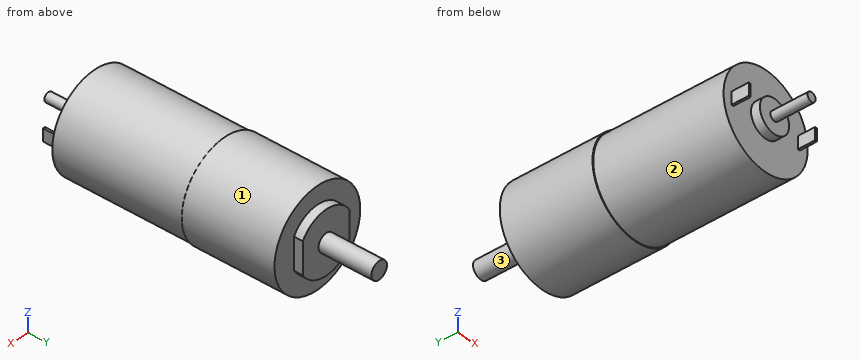
from build123d import *

# Parameters (mm, degrees)
SKETCH2_R           = 10.8
BOSS_EXTRUDE1_DEPTH = 29.5
SKETCH3_R           = 11
BOSS_EXTRUDE2_DEPTH = 21
BOSS_EXTRUDE3_DEPTH = 2
SKETCH5_R           = 2
BOSS_EXTRUDE4_DEPTH = 12
SKETCH6_R           = 3.75
BOSS_EXTRUDE5_DEPTH = 2
SKETCH7_W           = 0.5
SKETCH7_H           = 2.8
BOSS_EXTRUDE6_DEPTH = 3.9
SKETCH8_R           = 1.05
BOSS_EXTRUDE7_DEPTH = 8.4


with BuildPart() as part:
    # Sketch2 → Boss-Extrude1 (new body)
    with BuildSketch(Plane(origin=(0, 0, 0), x_dir=(1, 0, 0), z_dir=(0, 1, 0))):
        with Locations(Location((0, 0, 0), (0, 0, 270))):
            Circle(SKETCH2_R)
    extrude(amount=BOSS_EXTRUDE1_DEPTH)

    # Sketch3 → Boss-Extrude2 (add)
    with BuildSketch(Plane(origin=(0, 29.5, 0), x_dir=(1, 0, 0), z_dir=(0, 1, 0))):
        with Locations(Location((0, 0, 0), (0, 0, 90))):
            Circle(SKETCH3_R)
    extrude(amount=BOSS_EXTRUDE2_DEPTH)

    # Sketch4 → Boss-Extrude3 (add)
    with BuildSketch(Plane(origin=(0, 50.5, 0), x_dir=(1, 0, 0), z_dir=(0, 1, 0))):
        with BuildLine():
            Line((6, 3.605551275), (6, -3.605551275))
            ThreePointArc((6, -3.605551275), (0, -7), (-6, -3.605551275))
            Line((-6, -3.605551275), (-6, 3.605551275))
            ThreePointArc((-6, 3.605551275), (0, 7), (6, 3.605551275))
        make_face()
    extrude(amount=BOSS_EXTRUDE3_DEPTH)

    # Sketch5 → Boss-Extrude4 (add)
    with BuildSketch(Plane(origin=(0, 52.5, 0), x_dir=(1, 0, 0), z_dir=(0, 1, 0))):
        with Locations(Location((0, 0, 0), (0, 0, 270))):
            Circle(SKETCH5_R)
    extrude(amount=BOSS_EXTRUDE4_DEPTH)

    # Sketch6 → Boss-Extrude5 (add)
    with BuildSketch(Plane.XZ):
        with Locations(Location((0, 0, 0), (0, 0, 270))):
            Circle(SKETCH6_R)
    extrude(amount=BOSS_EXTRUDE5_DEPTH)

    # Sketch7 → Boss-Extrude6 (add)
    with BuildSketch(Plane.XZ):
        with Locations((-8.5, 0)):
            Rectangle(SKETCH7_W, SKETCH7_H)
        with Locations((8.5, 0)):
            Rectangle(SKETCH7_W, SKETCH7_H)
    extrude(amount=BOSS_EXTRUDE6_DEPTH)

    # Sketch8 → Boss-Extrude7 (add)
    with BuildSketch(Plane.XZ.offset(2)):
        with Locations(Location((0, 0, 0), (0, 0, 270))):
            Circle(SKETCH8_R)
    extrude(amount=BOSS_EXTRUDE7_DEPTH)


solid = part.part
Could you check a few things on this model? Use its own coordinates, in mm. Face numbers are marked on the shaded views. A direction names the side the tool comes from. Give positions to 0.01 mm unless a question says otherwise; leave off trailing zeros. Write each loop counter-clockwise with the first axis right and the second up, starting at its lowest first coordinate (ties: lowest second). Pieces come first, ordered by that corner, then holes. Notation, with made-up numbers: (10, 82.25) -> (45, 82.25) arc R22 cw to (45, 89.25) -> close; hole circle Ø7 at (60.25, 79.25). An arc over 180 degrees is marked (long way). Answer as CSV lines item,"result". Start each with the question number.
(1) Which directions (+Z, -Z, +X, -X, +Y, -Y) give clear straight access to the entire face, cutting with the end or side of a thin tool? Please do the marked faces 1, 2 and 3.
(2) I'm going to push flat-ended pins straight in: pin 1 Ø0.8 at (y, z) = (-2.5, 0) entering from -X; pin 2 Ø12 at (y, z) = (21, -4) entering from -X; pin 3 Ø0.8 at (y, z) = (-2, 0) entering from +X. Where does each tip first touch, or does it pass through?
(3) If we section it at D-D, the plane x = 9.75: Write out the boundary of the cut face in (y, z), and give its area (3 significant figures).
(4) Please list where these lines run through material, in increasing order: line 1 (X direction, y = -1.5, z = -0.25); line 2 (X direction, y = 28, z = -0.5); line 3 (Y direction, x = 9.5, z = 4.5).
(5) If we section it at B-B, the plane x = 0: Write out the boundary of the cut face in (y, z), and give its area (3 significant figures).
(6) If we section it at C-C, the plane y = 21: Write out the boundary of the cut face in (x, z), and give its area (3 significant figures).
Answer list:
1,face 1,"+Y, -Y"
1,face 2,"-Y"
1,face 3,"+Y"
2,pin 1,"x = -8.75"
2,pin 2,"x = -10.8"
2,pin 3,"x = 8.75"
3,outline,"(0, -4.65) -> (29.5, -4.65) -> (29.5, -5.09) -> (50.5, -5.09) -> (50.5, 5.09) -> (29.5, 5.09) -> (29.5, 4.65) -> (0, 4.65) -> close"
3,area,"488 mm^2"
4,line 1,"-8.75 to -8.25, -3.74 to 3.74, 8.25 to 8.75"
4,line 2,"-10.79 to 10.79"
4,line 3,"0 to 50.5"
5,outline,"(-10.4, -1.05) -> (-2, -1.05) -> (-2, -3.75) -> (0, -3.75) -> (0, -10.8) -> (29.5, -10.8) -> (29.5, -11) -> (50.5, -11) -> (50.5, -7) -> (52.5, -7) -> (52.5, -2) -> (64.5, -2) -> (64.5, 2) -> (52.5, 2) -> (52.5, 7) -> (50.5, 7) -> (50.5, 11) -> (29.5, 11) -> (29.5, 10.8) -> (0, 10.8) -> (0, 3.75) -> (-2, 3.75) -> (-2, 1.05) -> (-10.4, 1.05) -> close"
5,area,"1,210 mm^2"
6,outline,"circle Ø21.6 at (0, 0)"
6,area,"366 mm^2"
